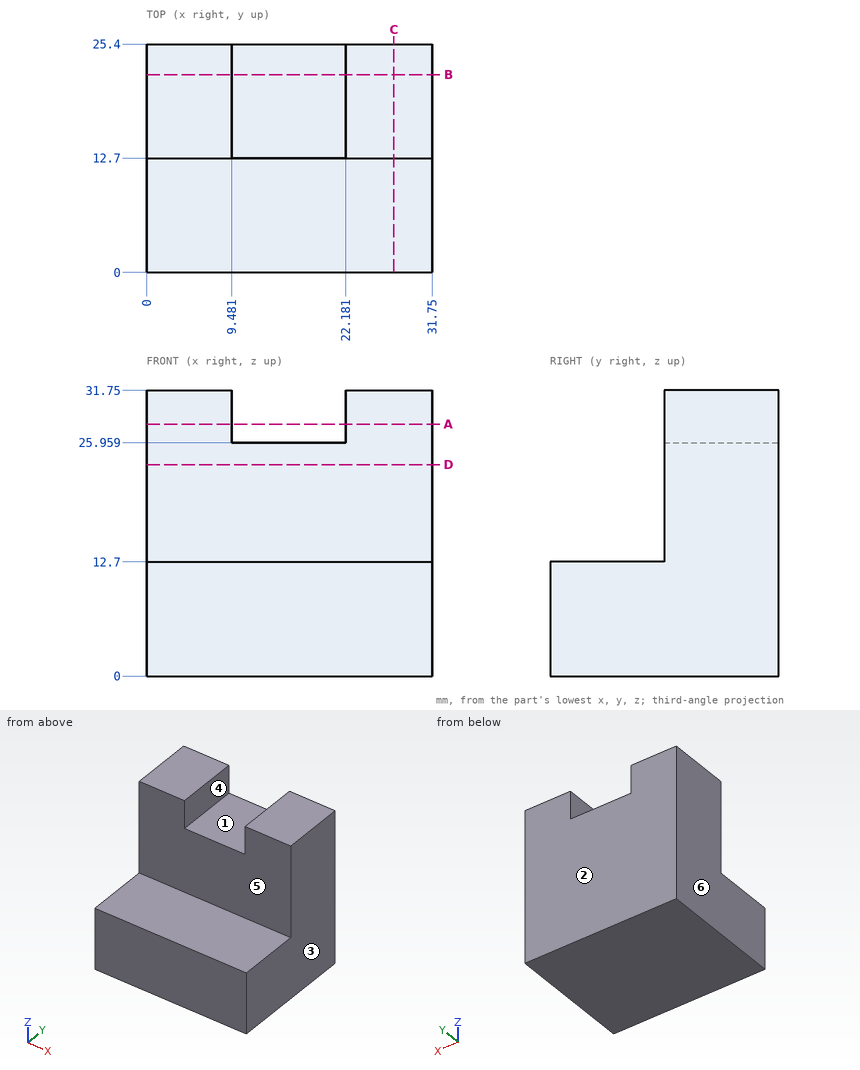
Input: dimensioned drawing with shaded views. Units: mm. Origin: part minimum x, y, z. A direction names the side the tool comes from. Give positions to 0.01 mm unless a question says otherwise; leave off trailing zeros. Order: outer loops, then holes, each group sorted by start corner. A loop starts at its lowest first (then second) coordinate and runs counter-clockwise, first axis right, second up.
(1) Section query B-B (y = 22). Return the cut outline in (x, z).
(2) Section query A-A (z = 28). Return the cut outline in (x, y).
(3) Pull-direction query (X, two-part tool) for the marked faces 1, 2, 3 and 4; classes: +X half, -X half, draft (parallel to the pull), parting line (faces both ways), or undercut.
(4) Contact query for flat-ended pins moving along their axis: P1, Ø3, axis at y = 19, z = 29, coming from the -X side; P2, Ø5.5, axis at x = 10, z = 27, coming from the -Y side. Output: stop coordinate, or through.
(5) Material intervals for line 1 along X through (y, z) = (22.5, 29.5); line 2 along Z through (x, y) = (9, 2); line 3 along Y through (x, z) = (30, 13), sorted ascending.
(6) Access query for the marked faces 5 and 6. Directions: +Z, -Z, +X, -X, +Y, -Y. A direction counts if a zero-diameter tool reaches every point of the face in a straight line with its end or side. Return the directions, or none.
(7) Section query C-C (x = 27.5). Return the cut outline in (y, z).
(8) Section query D-D (z = 23.5). Return the cut outline in (x, y), plus the area to 3 significant figures.
Outcome:
1. outline: (0, 0) - (31.75, 0) - (31.75, 31.75) - (22.18, 31.75) - (22.18, 25.96) - (9.48, 25.96) - (9.48, 31.75) - (0, 31.75) - close
2. outline: (0, 12.7) - (9.48, 12.7) - (9.48, 25.4) - (0, 25.4) - close; (22.18, 12.7) - (31.75, 12.7) - (31.75, 25.4) - (22.18, 25.4) - close
3. face 1: undercut
3. face 2: draft
3. face 3: +X half
3. face 4: undercut
4. P1: stops at x = 0
4. P2: stops at y = 12.7
5. line 1: x = 0 to 9.48, 22.18 to 31.75
5. line 2: z = 0 to 12.7
5. line 3: y = 12.7 to 25.4
6. face 5: +Z, +X, -X, -Y
6. face 6: +Z, -Z, -X, +Y, -Y
7. outline: (0, 0) - (25.4, 0) - (25.4, 31.75) - (12.7, 31.75) - (12.7, 12.7) - (0, 12.7) - close
8. outline: (0, 12.7) - (31.75, 12.7) - (31.75, 25.4) - (0, 25.4) - close
8. area: 403 mm2
